Can you work these out from the model? Positions are in its coordinate system, mm. Face numbers are marked on the shaded views. A direction names the side the tool comes from. Round coordinates to 2 decimals unless told otherwise and drop trailing zeros. Loops run counter-clockwise (first coordinate to the right, second up) from the corner with the lowest first, then second, coordinate; pieces in that order, holes last.
```python
from build123d import *

# Parameters (mm, degrees)
SKETCH1_W                 = 11.5344
SKETCH1_H                 = 77.978
BOSS_EXTRUDE1_DEPTH       = 6.35
F_4_40_TAPPED_HOLE1_D     = 2.2606
F_4_40_TAPPED_HOLE1_DEPTH = 6.35
F_4_40_TAPPED_HOLE1_TIP   = 0.679152758
SKETCH2_W                 = 9.5344
SKETCH2_H                 = 38.3286
SKETCH2_W_2               = 7.56565
SKETCH2_H_2               = 15.4178
CUT_EXTRUDE1_DEPTH        = 40.921488159
SKETCH8_W                 = 5
SKETCH8_H                 = 6.35
CUT_EXTRUDE2_DEPTH        = 40.921488159
SKETCH9_W                 = 6.5344
SKETCH9_H                 = 7
BOSS_EXTRUDE2_DEPTH       = 6.35
F_4_40_TAPPED_HOLE2_D     = 2.2606
F_4_40_TAPPED_HOLE2_DEPTH = 5
F_4_40_TAPPED_HOLE2_TIP   = 0.679152758
SKETCH10_W                = 3
SKETCH10_H                = 49.7694
BOSS_EXTRUDE3_DEPTH       = 6.35
FILLET1_R                 = 3.175


with BuildPart() as part:
    # Sketch1 → Boss-Extrude1 (new body)
    with BuildSketch(Plane(origin=(0, 0, 0), x_dir=(1, 0, 0), z_dir=(0, 1, 0))):
        Rectangle(SKETCH1_W, SKETCH1_H)
    extrude(amount=BOSS_EXTRUDE1_DEPTH)

    # #4-40 Tapped Hole1
    with Locations(Plane(origin=(5.7672, 0, 0), x_dir=(0, 0, -1), z_dir=(1, 0, 0))):
        with Locations((34.5186, 3.175), (-12.7508, 3.175)):
            Hole(F_4_40_TAPPED_HOLE1_D / 2, depth=F_4_40_TAPPED_HOLE1_DEPTH)
            with Locations((0, 0, -(F_4_40_TAPPED_HOLE1_DEPTH + F_4_40_TAPPED_HOLE1_TIP / 2))):  # 118° drill point
                Cone(0, F_4_40_TAPPED_HOLE1_D / 2, F_4_40_TAPPED_HOLE1_TIP, mode=Mode.SUBTRACT)

    # Sketch2 → Cut-Extrude1 (cut, through all)
    with BuildSketch(Plane(origin=(0, 6.35, 0), x_dir=(1, 0, 0), z_dir=(0, 1, 0))):
        with Locations((1, 10.8839)):
            Rectangle(SKETCH2_W, SKETCH2_H)
        with Locations((1.984375, -24.9301)):
            Rectangle(SKETCH2_W_2, SKETCH2_H_2)
    extrude(amount=-CUT_EXTRUDE1_DEPTH, mode=Mode.SUBTRACT)

    # Sketch8 → Cut-Extrude2 (cut, through all)
    with BuildSketch(Plane(origin=(0, 6.35, 0), x_dir=(1, 0, 0), z_dir=(0, 1, 0))):
        with Locations((3.2672, -35.814)):
            Rectangle(SKETCH8_W, SKETCH8_H)
    extrude(amount=-CUT_EXTRUDE2_DEPTH, mode=Mode.SUBTRACT)

    # Sketch9 → Boss-Extrude2 (add)
    with BuildSketch(Plane.XY.offset(38.989)):
        with Locations((-2.5, -3.5)):
            Rectangle(SKETCH9_W, SKETCH9_H)
    extrude(amount=-BOSS_EXTRUDE2_DEPTH)

    # #4-40 Tapped Hole2
    with Locations(Plane.XY.offset(38.989)):
        with Locations((-2.5, 2.85), (-2.5, -3.5)):
            Hole(F_4_40_TAPPED_HOLE2_D / 2, depth=F_4_40_TAPPED_HOLE2_DEPTH)
            with Locations((0, 0, -(F_4_40_TAPPED_HOLE2_DEPTH + F_4_40_TAPPED_HOLE2_TIP / 2))):  # 118° drill point
                Cone(0, F_4_40_TAPPED_HOLE2_D / 2, F_4_40_TAPPED_HOLE2_TIP, mode=Mode.SUBTRACT)

    # Sketch10 → Boss-Extrude3 (add)
    with BuildSketch(Plane.XZ):
        with Locations((-7.2672, -14.1043)):
            Rectangle(SKETCH10_W, SKETCH10_H)
    extrude(amount=-BOSS_EXTRUDE3_DEPTH)

    # Fillet1
    fillet1_edges = [part.edges().sort_by_distance(p)[0] for p in [
        (-3.782825, 0, 32.639),
    ]]
    fillet(fillet1_edges, radius=FILLET1_R)


solid = part.part
```
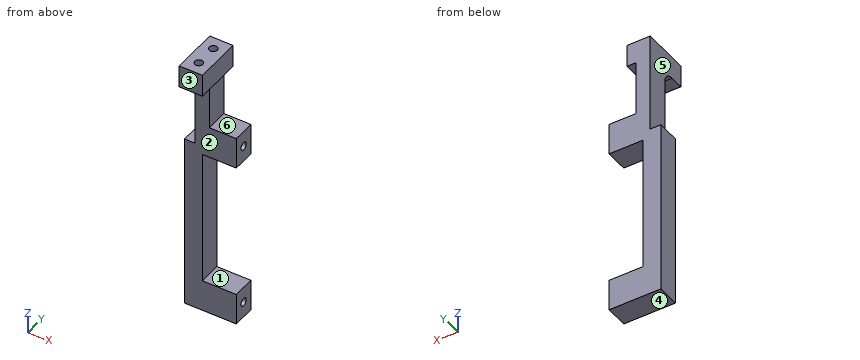
(1) If I drill on line 1 (Y direction, x = -2.5, z = 36.3); line 2 (Z direction, x = -1.25, y = 1.25); line 3 (X direction, y = 2.85, z = 35.3), over which ranges is the centre line in solid material (lowest first)?
(2) Suppose I cut it at A-A (z = 18). Write out the boundary of the cut face in (x, y), then the cut area to 3 significant figures.
(3) Suppose I cut it at B-B (y = -6). Write out the boundary of the cut face in (x, z), then the cut area to 3 significant figures.
(4) For pin 1 (3 mm diameter, centred on x = -0.5, z = -31, fed in from -Y); pin 2 (5 mm diameter, centred on y = 2, z = -5, fed in from +X); pin 3 (1 mm diameter, centred on y = -1, z = -15.5, fed in from -X); pin 4 (1.9 mm diameter, centred on y = 3, z = 35, fed in from +X), each with a flat end and sliding along its axis, tell me the tip position at first contact or that it passes through.
(5) We'd pull the mould along Z, two halves only. Please class the marked faces 4, 5 and 6: released by +Z, released by -Z, zero draft, split by the parting line, or undercut.
(6) Which directions (+Z, -Z, +X, -X, +Y, -Y) give clear straight access to the entire face, cutting with the end or side of a thin tool? Please do the marked faces 1, 2 and 3.
Check result:
1. line 1: y = -7 to -4.63, -2.37 to 1.72, 3.98 to 6.35
1. line 2: z = -38.99 to -30.05, 8.28 to 17.22, 32.64 to 38.99
1. line 3: x = -5.77 to -3.63, -1.37 to 0.77
2. outline: (-5.77, 0) - (-1.8, 0) - (-1.8, 6.35) - (-5.77, 6.35) - close
2. area: 25.2 mm2
3. outline: (-5.77, 32.64) - (0.77, 32.64) - (0.77, 38.99) - (-5.77, 38.99) - close
3. area: 41.5 mm2
4. pin 1: stops at y = 0
4. pin 2: stops at x = -3.77
4. pin 3: passes through
4. pin 4: stops at x = 0.77
5. face 4: released by -Z
5. face 5: zero draft
5. face 6: undercut
6. face 1: +X, +Y, -Y
6. face 2: -Z, +X, -X, -Y
6. face 3: +Z, -Z, +X, -X, -Y
